from build123d import *

# Parameters (mm, degrees)
F0_R     = 40
F0_R_2   = 29
F1_DEPTH = 2


with BuildPart() as f1:
    # F0 (on Top) → F1 (new body)
    with BuildSketch(Plane.XY):
        Circle(F0_R)
        Circle(F0_R_2, mode=Mode.SUBTRACT)
    extrude(amount=F1_DEPTH)

    # F2 (on Front) → F3 (revolve)
    with BuildSketch(Plane.XZ):
        Polygon((31.969388, 5), (28.969388, 2), (31.969388, 2), (33.469388, 2), (33.469388, 5), align=None)
    revolve(axis=Axis((0, 0, 4.160745), (0, 0, 1)))


solid = f1.part
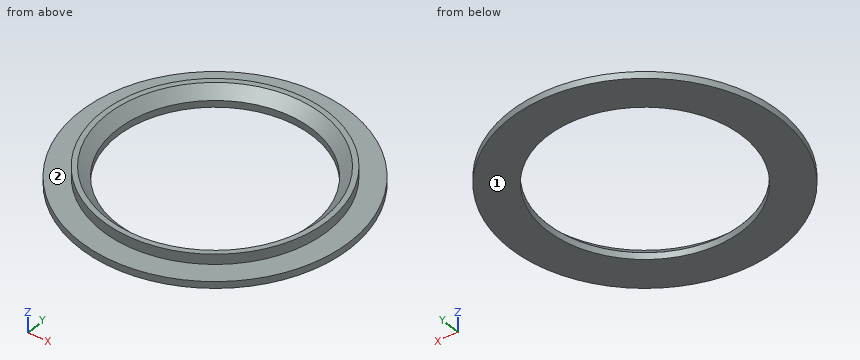
Check sheet for the modelled part. Datum: model origin and axes. Units: mm. Face numbers are marked on the shaded views. A direction names the side the tool comes from. Give positions to 0.01 mm unless a question says otherwise; leave off trailing zeros. Loops run counter-clockwise (first coordinate to the right, second up) from the corner with the lowest first, then second, coordinate; pieces in that order, holes last. Notation, with made-up numbers: M -37.5,21.25 L -8.5,21.25 A30 cw -8.5,48.25 Z; hole C -1.5,8 d2. An arc over 180 degrees is marked long. Answer as a JSON object with one key per item and string values. Group by question number.
Q1. Access from +Z, -Z, +X, -X, +Y, -Y to the whole of each face (thin tool, end or side, straight path). Record for the marked faces 1 and 2.
Q2. Go/stop test with flat-tipped pins: P1, Ø1.5, axis at x = -14.5, z = 3.5, coming from the +Y side; P2, Ø10, axis at x = -13, y = 20.5, coming from the +Z side; P3, Ø1.5, axis at x = -15.5, z = 4, coming from the +Y side. Record where each tip stops, or that it passes through.
Q3. Cross-section at C-C on z = 1.25. Record the cut outline in (x, y), then the cut area to 3 significant figures.
Q4. Material ranges on line 1 along Y through (x, z) = (0, 1.5); line 2 along X through (y, z) = (-22, 4.7); line 3 along X through (y, z) = (8, 2.3), recorded low to high. Write a range as [from, to].
Evaluation:
{
 "1": {"face 1": "-Z, +X, -X, +Y, -Y", "face 2": "+Z"},
 "2": {"P1": "stops at y = 30.51", "P2": "stops at z = 2.31", "P3": "stops at y = 30.04"},
 "3": {"outline": "C 0,0 d80; hole C 0,0 d58", "area": "2,380 mm2"},
 "4": {"line 1": "y = [-40, -29], [29, 40]", "line 2": "x = [-25.22, -22.78], [22.78, 25.22]", "line 3": "x = [-32.5, -28.15], [28.15, 32.5]"}
}
